Source: CAD feature listing. Evaluate the final solid. Frame: model axes, mm. Coordinates: 2 decimals unless noted, no trailing zeros. Write each loop counter-clockwise with the first axis right and the second up, starting at its lowest first coordinate (ties: lowest second). Pieces come first, ordered by that corner, then holes. Notation, with made-up numbers: M -11,-27 L 28,-27 A3 cw 28,-23 Z; hole C -6.5,-32 d1. An arc over 180 degrees is marked long. One line per item, written item: value. Start each with the question number.
Item 1: Cut plane A-A, the plane y = 27. Output: boundary loops of the cut face in (x, z).
Item 2: Mould query, pull axis Y, two halves, no side actions, for faces 1 (the flat face through (0, 35, 1)), 2 (the cylindrical face through (11.67, 29.48, 1.52)), 3 (the flat face through (0, 0, 3)). Classes: released by +Y, released by -Y, zero draft, split by the parting line, or undercut.
Item 3: Cut plane C-C, the plane x = -12. Output: boundary loops of the cut face in (y, z).
Item 4: Pin query (flat end, axial travel): P1, Ø3.5, axis at x = -12, y = -27, coming from the +Z side; P2, Ø4.5, axis at x = 12, y = 27, coming from the +Z side. Return the tip coordinate at first contact, or that it passes through.
Item 5: Ray query, L1, parallel to Y at x = 12, z = 0.85; L2, parallel to Y at x = -10, z = 0.75. Return the intervals inside material, ascending. Write a range as from..to.
Item 6: Cut plane D-D, the plane y = -13. Output: boundary loops of the cut face in (x, z), then the cut area to 3 significant figures.
Item 7: Cut plane B-B, the plane z = 0.85. State how many separate pieces and enclosed holes the cut face has, then the cut area to 3 significant figures.
```python
from build123d import *

# Parameters (mm, degrees)
EXTRUDE_1_DEPTH     = 3
SKETCH_2_R          = 1.55
CUT_EXTRUDE_1_DEPTH = 73.862884928
SKETCH_3_R          = 1.5
SKETCH_3_R_2        = 2.5
CUT_EXTRUDE_2_DEPTH = 73.862884928
SKETCH_4_W          = 40
SKETCH_4_H          = 35
CUT_EXTRUDE_3_DEPTH = 73.862884928


with BuildPart() as part:
    # 草图1 → 凸台-拉伸1 (new body)
    with BuildSketch(Plane.XY):
        Polygon((-20, 35), (0, 70), (20, 70), (20, 35), (20, -35), (-20, -35), align=None)
    extrude(amount=EXTRUDE_1_DEPTH)

    # 草图2 → 切除-拉伸1 (cut, through all)
    with BuildSketch(Plane.XY.offset(3)):
        with Locations((17, 61)):
            Circle(SKETCH_2_R)
        with Locations((6, 61)):
            Circle(SKETCH_2_R)
        with Locations((17, 41)):
            Circle(SKETCH_2_R)
        with Locations((4.851224059, 41)):
            Circle(SKETCH_2_R)
    extrude(amount=-CUT_EXTRUDE_1_DEPTH, mode=Mode.SUBTRACT)

    # 草图3 → 切除-拉伸2 (cut, through all)
    with BuildSketch(Plane.XY.offset(3)):
        with Locations((12, -27)):
            Circle(SKETCH_3_R)
        with Locations((-12, -27)):
            Circle(SKETCH_3_R)
        with Locations((12, -13)):
            Circle(SKETCH_3_R)
        with Locations((-12, -13)):
            Circle(SKETCH_3_R)
        with Locations((12, 3)):
            Circle(SKETCH_3_R_2)
        with Locations((-12, 3)):
            Circle(SKETCH_3_R_2)
        with Locations((12, 27)):
            Circle(SKETCH_3_R_2)
        with Locations((-12, 27)):
            Circle(SKETCH_3_R_2)
    extrude(amount=-CUT_EXTRUDE_2_DEPTH, mode=Mode.SUBTRACT)

    # 草图4 → 切除-拉伸3 (cut, through all)
    with BuildSketch(Plane(origin=(0, 0, 0), x_dir=(-1, 0, 0), z_dir=(0, 0, -1))):
        with Locations((0, 52.5)):
            Rectangle(SKETCH_4_W, SKETCH_4_H)
    extrude(amount=-CUT_EXTRUDE_3_DEPTH, mode=Mode.SUBTRACT)


solid = part.part
```
From the geometry:
1. outline: M -20,0 L -14.5,0 L -14.5,3 L -20,3 Z; M -9.5,0 L 9.5,0 L 9.5,3 L -9.5,3 Z; M 14.5,0 L 20,0 L 20,3 L 14.5,3 Z
2. face 1: released by +Y
2. face 2: undercut
2. face 3: zero draft
3. outline: M -35,0 L -28.5,0 L -28.5,3 L -35,3 Z; M -25.5,0 L -14.5,0 L -14.5,3 L -25.5,3 Z; M -11.5,0 L 0.5,0 L 0.5,3 L -11.5,3 Z; M 5.5,0 L 24.5,0 L 24.5,3 L 5.5,3 Z; M 29.5,0 L 35,0 L 35,3 L 29.5,3 Z
4. P1: stops at z = 3
4. P2: passes through
5. L1: y = -35..-28.5, -25.5..-14.5, -11.5..0.5, 5.5..24.5, 29.5..35
5. L2: y = -35..1.5, 4.5..25.5, 28.5..35
6. outline: M -20,0 L -13.5,0 L -13.5,3 L -20,3 Z; M -10.5,0 L 10.5,0 L 10.5,3 L -10.5,3 Z; M 13.5,0 L 20,0 L 20,3 L 13.5,3 Z
6. area: 102 mm²
7. separate pieces: 1
7. enclosed holes: 8
7. area: 2,690 mm²
